from build123d import *

# Parameters (mm, degrees)
WALL_DEPTH                = 19.05
ROOF_START                = 19.05
ROOF_DEPTH                = 3.175
F_2_56_TAPPED_HOLE1_D     = 1.778
F_2_56_TAPPED_HOLE1_DEPTH = 5.73
F_2_56_TAPPED_HOLE1_TIP   = 0.53416509
F_2MM_DEPTH_CUT_DEPTH     = 2
F_1_16_IN_FILLET_R        = 1.5875


with BuildPart() as part:
    # MainSketch → Wall (new body)
    with BuildSketch(Plane(origin=(0, 0, 0), x_dir=(1, 0, 0), z_dir=(0, 1, 0))):
        Polygon((-32.75, -4), (0, -4), (0, 0), (-36.75, 0), (-36.75, -45.5), (0, -45.5), (0, -41.5), (-32.75, -41.5), align=None)
    extrude(amount=WALL_DEPTH)

    # MainSketch<3> → Roof (add)
    with BuildSketch(Plane(origin=(0, 0, 0), x_dir=(1, 0, 0), z_dir=(0, 1, 0)).offset(ROOF_START)):
        with BuildLine():
            Line((0, -21.625), (0, 0))
            Line((0, 0), (-36.75, 0))
            Line((-36.75, 0), (-36.75, -45.5))
            Line((-36.75, -45.5), (0, -45.5))
            Line((0, -45.5), (0, -23.875))
            ThreePointArc((0, -23.875), (-0.353553391, -23.728553391), (-0.5, -23.375))
            Line((-0.5, -23.375), (-0.5, -22.125))
            ThreePointArc((-0.5, -22.125), (-0.353553391, -21.771446609), (0, -21.625))
        make_face()
    extrude(amount=ROOF_DEPTH)

    # #2-56 Tapped Hole1
    with Locations(Plane(origin=(-18.375, 0, 2.5), x_dir=(0, 0, -1), z_dir=(0, -1, 0))):
        with Locations((0, 0), (-40.5, 0)):
            Hole(F_2_56_TAPPED_HOLE1_D / 2, depth=F_2_56_TAPPED_HOLE1_DEPTH)
            with Locations((0, 0, -(F_2_56_TAPPED_HOLE1_DEPTH + F_2_56_TAPPED_HOLE1_TIP / 2))):  # 118° drill point
                Cone(0, F_2_56_TAPPED_HOLE1_D / 2, F_2_56_TAPPED_HOLE1_TIP, mode=Mode.SUBTRACT)

    # Sketch3 → 2mm depth cut (cut)
    with BuildSketch(Plane(origin=(0, 0, 0), x_dir=(0, 0, -1), z_dir=(1, 0, 0))):
        Polygon((-44.25, 21.3875), (-44.25, 0), (-42.75, 0), (-42.75, 19.8875), (-24.875, 19.8875), (-24.875, 21.3875), align=None)
        Polygon((-1.25, 21.3875), (-20.625, 21.3875), (-20.625, 19.8875), (-2.75, 19.8875), (-2.75, 0), (-1.25, 0), align=None)
    extrude(amount=-F_2MM_DEPTH_CUT_DEPTH, mode=Mode.SUBTRACT)

    # 1/16 in fillet
    f_1_16_in_fillet_edges = [part.edges().sort_by_distance(p)[0] for p in [
        (-1, 19.8875, 42.75),
        (-1, 21.3875, 44.25),
        (-2, 20.6375, 24.875),
        (-1, 21.3875, 1.25),
        (-1, 19.8875, 2.75),
        (-2, 20.6375, 20.625),
    ]]
    fillet(f_1_16_in_fillet_edges, radius=F_1_16_IN_FILLET_R)


solid = part.part
Geometry: final body of the model. Coordinates: model frame, mm. A direction names the side the tool comes from. Give positions to 0.01 mm unless a question says otherwise; leave off trailing zeros. Order: outer loops, then holes, each group sorted by start corner. A loop starts at its lowest first (then second) coordinate and runs counter-clockwise, first axis right, second up. Notation, with made-up numbers: (55, 45) -> (72, 45) arc R22 ccw to (72, 78) -> close; hole circle Ø8 at (21, 56.25). An arc over 180 degrees is marked (long way). Put each result on its own line as item: value.
Q1. Draft query along Y for faces 1 (the face through (-33, 0, 23)), 2 (the face through (-1, 21.388, 12)), 3 (the face through (-1, 19.888, 13)), 4 (the face through (-16, 9, 41.5)). Return one class per face: released by +Y, released by -Y, zero draft, split by the parting line, or undercut.
Here are the results:
face 1: released by -Y
face 2: undercut
face 3: undercut
face 4: zero draft
Q2. Reachability of faces 5 (the face through (-0.5, 21, 23)), 6 (the face through (-1.01, 19.41, 3.2)), 7 (the face through (-17.494, 2.905, 2.384)), 8 (the face through (-17, 9, 4)) from +Z, -Z, +X, -X, +Y, -Y: full face, straight path, thin tool, end or side. Return the list, or none.
Here are the results:
face 5: +X, +Y, -Y
face 6: +X
face 7: -Y
face 8: +X, -Y
Q3. Section B-B, the plane y = 8.5. Return loops of the section in (x, z).
Here are the results:
outline: (-36.75, 0) -> (0, 0) -> (0, 1.25) -> (-2, 1.25) -> (-2, 2.75) -> (0, 2.75) -> (0, 4) -> (-32.75, 4) -> (-32.75, 41.5) -> (0, 41.5) -> (0, 42.75) -> (-2, 42.75) -> (-2, 44.25) -> (0, 44.25) -> (0, 45.5) -> (-36.75, 45.5) -> close
Q4. Material intervals for L1, parallel to Z at x = -7, y = 11.75; L2, parallel to X at y = 4.1, z = 2.5; L3, parallel to Y at x = -21, z = 5 (3 decimals), sorted ascending.
Here are the results:
L1: z = 0 to 4, 41.5 to 45.5
L2: x = -36.75 to -19.26, -17.49 to -2
L3: y = 19.05 to 22.225
Q5. Pin query (flat end, axial travel): pin 1 (8 mm diameter, centred on x = -4, z = 32, fed in from -Y). Return the tip coordinate at first contact, or that it passes through.
Here are the results:
pin 1: stops at y = 19.05
Q6. Section A-A, the plane x = -24.5. Return loops of the section in (y, z) (3 decimals), then the cut area to 3 significant figures.
Here are the results:
outline: (0, 0) -> (22.225, 0) -> (22.225, 45.5) -> (0, 45.5) -> (0, 41.5) -> (19.05, 41.5) -> (19.05, 4) -> (0, 4) -> close
area: 297 mm^2
